Could you check a few things on this model? Use its own coordinates, in mm. Face numbers are marked on the shaded views. A direction names the side the tool comes from. Coordinates: 2 decimals unless noted, no trailing zeros. Write each loop counter-clockwise with the first axis right and the second up, starting at its lowest first coordinate (ties: lowest second). Pieces come first, ordered by that corner, then holes.
Item 1: If I drill on probe 1 along Z at (x, y) = (0, 16.95); probe 2 along X at (y, z) = (17.9, -24.5); probe 3 along X at (y, z) = (5.75, 7), over which ranges is the centre line in solid material (lowest first)?
Item 2: I want a section at D-D on x = -20. Please give me the cut outline in (y, z).
Item 3: I want a section at A-A on z = -24.5. Please give me the cut outline in (x, y).
Item 4: For P1, Ø5.5, axis at x = -3, z = -7, coming from the +Y side; P2, Ø2, axis at x = -16.5, y = 18.5, coming from the -Z side; P3, Ø3, axis at y = 6, z = -9, coming from the -X side, each with a flat end and sliding along its axis, tell me the tip position at first contact or that it passes through.
Item 5: Which directions (+Z, -Z, +X, -X, +Y, -Y) give clear straight access to the entire face, cutting with the end or side of a thin tool? Please do the marked faces 1, 2 and 3.
Item 6: I want a section at B-B on y = 12. Please give me the cut outline in (x, z), then the cut area to 3 significant figures.
Item 7: I want a section at C-C on z = -13.5. Please give me the cut outline in (x, y), then the cut area to 3 significant figures.
Autodesk Inventor part; units mm, degrees
ref_plane "YZ Plane" through (0, 0, 0) normal (1, 0, 0) x (0, 1, 0)
ref_plane "XZ Plane" through (0, 0, 0) normal (0, 1, 0) x (-1, 0, 0)
ref_plane "XY Plane" through (0, 0, 0) normal (0, 0, 1) x (1, 0, 0)
sketch "Esboço1" plane through (0, 0, 0) normal (0, 1, 0) x (-1, 0, 0)
  line L0 (-12, 17) -> (12, 17)
  line L1 (12, 17) -> (12, -17)
  line L2 (12, -17) -> (-12, -17)
  line L3 (-12, -17) -> (-12, 17)
  line L4 (-12, 17) -> (12, -17) construction
  line L5 (12, 17) -> (-12, -17) construction
  point P0 (0, 0)
  dimension "d0" = 24
  dimension "d1" = 34
extrude "Extrusão1" add sketch "Esboço1" along normal blind 20
shell "Casca1" thickness 2 removed faces 1 at (4, 20, 5.6667)
sketch "Esboço2" plane through (-10, 2, 15) normal (0, 1, 0) x (1, 0, 0)
  line L0 (16, 8) -> (4, 8)
  line L1 (4, 8) -> (4, 25)
  line L2 (4, 25) -> (16, 25)
  line L3 (16, 25) -> (16, 8)
  line L4 (16, 8) -> (4, 25) construction
  line L5 (4, 8) -> (16, 25) construction
  line L6 (0, 30) -> (20, 30)
  circle A0 centre (6.5, 22.5) radius 1.5
  circle A1 centre (13.5, 22.5) radius 1.5
  point P0 (10, 15)
  point P1 (10, 16.5)
  dimension "d5" = 12
  dimension "d6" = 17
  dimension "d7" = 5
  dimension "d8" = 3
  dimension "d9" = 2.5
  dimension "d10" = 2.5
  dimension "d11" = 3
  dimension "d12" = 2.5
extrude "Extrusão2" cut sketch "Esboço2" against normal blind 30 contours A0 | A1
sketch "Esboço5" plane through (-10, 2, 15) normal (0, 1, 0) x (1, 0, 0)
  circle A0 centre (13.5, 22.5) radius 1.5
  arc A1 (11.65, 22.5) -> (15.35, 22.5) centre (13.5, 22.5) ccw
  circle A2 centre (13.5, 22.5) radius 1.5
  circle A3 centre (6.5, 22.5) radius 1.5
  circle A4 centre (6.5, 22.5) radius 1.5
  arc A5 (4.65, 22.5) -> (8.35, 22.5) centre (6.5, 22.5) ccw
  arc A6 (16.5, 22.5) -> (10.5, 22.5) centre (13.5, 22.5) ccw
  arc A7 (9.5, 22.5) -> (3.5, 22.5) centre (6.5, 22.5) ccw
  line L0 (15.35, 22.5) -> (16.5, 22.5)
  line L1 (11.65, 22.5) -> (10.5, 22.5)
  line L2 (8.35, 22.5) -> (9.5, 22.5)
  line L3 (3.5, 22.5) -> (4.65, 22.5)
  point P0 (10, 15)
  dimension "d32" = 3.7
  dimension "d33" = 3.7
  dimension "d34" = 6
  dimension "d35" = 6
extrude "Extrusão5" add sketch "Esboço5" along normal blind 0.8
sketch "Esboço6" plane through (-10, 2, 15) normal (0, 1, 0) x (1, 0, 0)
  circle A0 centre (10, 17) radius 4.1
  line L0 (16, 8) -> (4, 8)
  line L1 (4, 8) -> (4, 25)
  line L2 (4, 25) -> (16, 25)
  line L3 (16, 25) -> (16, 8)
  line L4 (16, 8) -> (4, 25) construction
  line L5 (4, 8) -> (16, 25) construction
  line L6 (0, 30) -> (20, 30)
  point P0 (10, 15)
  point P1 (10, 16.5)
  dimension "d38" = 8.2
  dimension "d39" = 12
  dimension "d40" = 17
  dimension "d41" = 5
  dimension "d42" = 9
extrude "Extrusão6" cut sketch "Esboço6" against normal blind 2 contours A0
sketch "Esboço8" plane through (0, 20, 0) normal (0, 1, 0) x (1, 0, 0)
  line L0 (-12, 17) -> (12, 17)
  line L1 (12, 17) -> (-12, 17)
  line L2 (-12, 17) -> (-12, 32)
  line L3 (-12, 32) -> (12, 32)
  line L4 (12, 32) -> (12, 17)
  line L5 (-12, -17) -> (-12, 17)
  line L6 (-12, -12) -> (-27, -12)
  line L7 (-27, -12) -> (-27, 12)
  line L8 (-27, 12) -> (-12, 12)
  line L9 (-12, 12) -> (-12, -12)
  point P0 (0, 0)
  dimension "d57" = 15
  dimension "d58" = 15
  dimension "d59" = 24
  dimension "d60" = 5
extrude "Extrusão8" add sketch "Esboço8" against normal blind 4
chamfer "Chanfro3" distance 5 angle 45 4 edges at (-27, 18, -12) (-12, 18, -32) (12, 18, -32) (-27, 18, 12)
sketch "Esboço9" plane through (0, 20, 0) normal (0, 1, 0) x (1, 0, 0)
  circle A0 centre (-19.5, 0) radius 2
  circle A1 centre (0, 24.5) radius 2
  line L0 (-27, 7) -> (-27, -7)
  line L1 (7, 32) -> (-7, 32)
  point P0 (0, 0)
  dimension "d66" = 4
  dimension "d67" = 4
  dimension "d68" = 7.5
  dimension "d69" = 7.5
extrude "Extrusão9" cut sketch "Esboço9" against normal blind 4
sketch "Esboço11" plane through (-12, 0, 17) normal (0, 0, 1) x (1, 0, 0)
  arc A0 (10, 11) -> (10, 7) centre (10, 9) ccw
  line L0 (24, 0) -> (0, 0)
  line L1 (0, 0) -> (0, 20)
  arc A1 (14, 7) -> (14, 11) centre (14, 9) ccw
  line L2 (24, 0) -> (24, 20)
  line L3 (10, 11) -> (14, 11)
  line L4 (14, 7) -> (10, 7)
  point P0 (12, 0)
  dimension "d79" = 4
  dimension "d80" = 9
  dimension "d81" = 10
  dimension "d82" = 4
  dimension "d83" = 10
extrude "Extrusão11" cut sketch "Esboço11" against normal blind 4
properties part number "Caixa mlx"
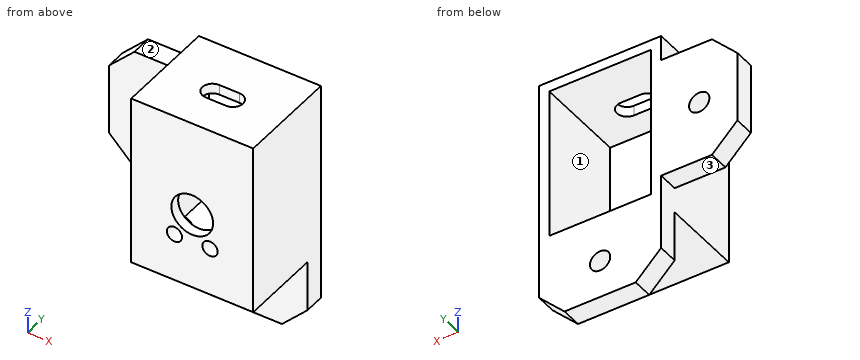
Response values:
1. probe 1: z = -32 to -26.5, -22.5 to -15, 15 to 17
1. probe 2: x = -12 to -2, 2 to 12
1. probe 3: x = -12 to -10, 10 to 12
2. outline: (16, -12) - (20, -12) - (20, -1.94) - (16, -1.94) - close; (16, 1.94) - (20, 1.94) - (20, 12) - (16, 12) - close
3. outline: (-12, 16) - (-2, 16) - (-2, 20) - (-12, 20) - close; (2, 16) - (12, 16) - (12, 20) - (2, 20) - close
4. P1: stops at y = 2.8
4. P2: stops at z = -12
4. P3: stops at x = -12
5. face 1: +Y
5. face 2: +Z, -X, +Y, -Y
5. face 3: -Z, -X, +Y, -Y
6. outline: (-12, -17) - (12, -17) - (12, 17) - (-12, 17) - close; hole (-10, -15) - (10, -15) - (10, 15) - (-10, 15) - close
6. area: 216 mm2
7. outline: (-12, 0) - (12, 0) - (12, 20) - (10, 20) - (10, 2) - (-10, 2) - (-10, 20) - (-12, 20) - close
7. area: 120 mm2
